from build123d import *

# Parameters (mm, degrees)
F0_W     = 160
F0_H     = 320
F0_R     = 3
F0_R_2   = 17.5
F1_DEPTH = 2.5


# Not quite as in the source:
# - a fillet or chamfer that OpenCascade refuses, or shapes differently, is made with other operations: its cross-section is extruded or revolved along the edge and cut away or added


with BuildPart() as f1:
    # F0 (on Front) → F1 (new body)
    with BuildSketch(Plane.XZ):
        with Locations((-1.8876045942, 29.6809725389)):
            Rectangle(F0_W, F0_H)
        with Locations((-1.8876045942, -95.3190274611)):
            Circle(F0_R, mode=Mode.SUBTRACT)
        with Locations((-1.8876045942, -10.3190274611)):
            Circle(F0_R_2, mode=Mode.SUBTRACT)
        with Locations((-1.8876045942, 49.6809725389)):
            Circle(F0_R_2, mode=Mode.SUBTRACT)
        with Locations((-1.8876045942, 154.6809725389)):
            Circle(F0_R, mode=Mode.SUBTRACT)
    extrude(amount=F1_DEPTH)

    # F2: chamfer of 4 on 2 edges, made by hand

    # F2_s1 → F2_t2 (revolve, cut)
    with BuildSketch(Plane.XY.offset(154.6809725389)):
        Polygon((1.1123954058, 1.5), (5.1123954058, -2.5), (1.1123954058, -2.5), align=None)
    revolve(axis=Axis((-1.8876045942, -2.5, 154.6809725389), (0, -1, 0)), mode=Mode.SUBTRACT)

    # F2_s3 → F2_t4 (revolve, cut)
    with BuildSketch(Plane.XY.offset(-95.3190274611)):
        Polygon((1.1123954058, 1.5), (5.1123954058, -2.5), (1.1123954058, -2.5), align=None)
    revolve(axis=Axis((-1.8876045942, -2.5, -95.3190274611), (0, -1, 0)), mode=Mode.SUBTRACT)


solid = f1.part
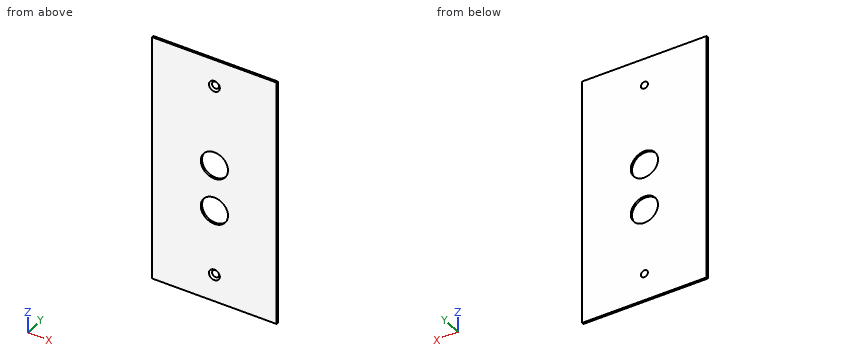
Can you work these out from the model? Positions are in its coordinate system, mm. Coordinates: 2 decimals unless noted, no trailing zeros. Write each loop counter-clockwise with the first axis right and the second up, starting at its lowest first coordinate (ties: lowest second). Pieces come first, ordered by that corner, then holes. Notation, with made-up numbers: (51.25, -29) -> (81.25, -29) arc R20 ccw to (81.25, 2) -> close; hole circle Ø10 at (-8, 11.5). An arc over 180 degrees is marked (long way). Write each question's results on one line, items separated by ' | '. Start each with the question number.
Item 1: Please list where these lines run through material, in increasing order: probe 1 along Z at (x, y) = (11, -0.55); probe 2 along Z at (x, y) = (10, -2); probe 3 along Z at (x, y) = (-5.5, -2.4).
Item 2: If we section it at A-A, the plane y = -1.65: Write out the boundary of the cut face in (x, z).
Item 3: If we section it at B-B, the plane x = -4: Count the separate pieces of the cut face and the enclosed holes in it, and give its area (3 significant figures).
Item 4: I'm going to push a flat-ended pin straight in: P1, Ø10, axis at x = -0.5, z = -41, coming from the +Y side. Where does the tip first touch, or does it pass through?
Answer block:
1) probe 1: -130.32 to -22.16, 1.52 to 37.84, 61.52 to 189.68 | probe 2: -130.32 to -23.16, 2.52 to 36.84, 62.52 to 189.68 | probe 3: -130.32 to -101.2, -89.44 to -27.44, 6.8 to 32.56, 66.8 to 148.8, 160.56 to 189.68
2) outline: (-81.89, -130.32) -> (78.11, -130.32) -> (78.11, 189.68) -> (-81.89, 189.68) -> close; hole circle Ø35 at (-1.89, -10.32); hole circle Ø35 at (-1.89, 49.68); hole circle Ø12.3 at (-1.89, -95.32); hole circle Ø12.3 at (-1.89, 154.68)
3) separate pieces: 5 | enclosed holes: 0 | area: 573 mm²
4) P1: y = 0
